Here's how the part is built. I have some questions about the finished solid (model axes, mm). A direction names the side the tool comes from. Coordinates: 2 decimals unless noted, no trailing zeros. Write each loop counter-clockwise with the first axis right and the second up, starting at its lowest first coordinate (ties: lowest second). Pieces come first, ordered by that corner, then holes.
(1) Which directions (+Z, -Z, +X, -X, +Y, -Y) give clear straight access to the entire face, cutting with the end or side of a thin tool? Please do faces 1 (the flat face through (0, 2.9, 2)), 2 (the flat face through (0, 10.9, 0)), 3 (the flat face through (-1.095, 0.937, 0.644)).
(2) Imagine slicing it at A-A, the plane x = 0. List the corners of the cut face in (y, z) for me (3 decimals).
(3) For pin 1 Ø0.8 at (x, z) = (0, 0.5) entering from -Y; pin 2 Ø2 at (y, z) = (6.5, -1) entering from +X; pin 3 Ø2 at (x, y) = (0.5, 6) entering from -Z, each with a flat end and sliding along its axis, tell me the tip position at first contact or that it passes through.
(4) Imagine slicing it at C-C, the plane x = 1.95. List the corners of the cut face in (y, z) for me, plus the area to 3 significant figures.
(5) Thinking about a two-plate mould opening in Z: for faces 4 (the cylindrical face through (-1.45, 6.72, -0.06)), 5 (the flat face through (-1.105, 0.937, -0.626)), 6 (the flat face through (0, 1, -1.27)), 7 (the flat face through (1.1, 0, 1.1)), which applies, released by +Z, released by -Z, zero draft, split by the parting line, or undercut?
(6) Imagine slicing it at B-B, the plane y = 7.5. List the corners of the cut face in (x, z) for me.
(7) Please list where these lines run through material, in increasing order: probe 1 along Y at (x, z) = (-0.2, -0.9); probe 2 along Y at (x, z) = (1.3, -1.3); probe 3 along Z at (x, y) = (0.4, 1.5).
```python
from build123d import *

# Parameters (mm, degrees)
SKETCH1_R           = 2.465
BOSS_EXTRUDE1_DEPTH = 2.9
SKETCH2_R           = 1.45
BOSS_EXTRUDE2_DEPTH = 8
CUT_EXTRUDE1_DEPTH  = 1.9
CHAMFER1_SIZE       = 0.25


with BuildPart() as part:
    # Sketch1 → Boss-Extrude1 (new body)
    with BuildSketch(Plane(origin=(0, 0, 0), x_dir=(1, 0, 0), z_dir=(0, 1, 0))):
        Circle(SKETCH1_R)
    extrude(amount=BOSS_EXTRUDE1_DEPTH)

    # Sketch2 → Boss-Extrude2 (add)
    with BuildSketch(Plane(origin=(0, 2.9, 0), x_dir=(1, 0, 0), z_dir=(0, 1, 0))):
        Circle(SKETCH2_R)
    extrude(amount=BOSS_EXTRUDE2_DEPTH)

    # Sketch3 → Cut-Extrude1 (cut)
    with BuildSketch(Plane.XZ):
        Polygon((0.733234842, -1.27), (1.466469684, 0), (0.733234842, 1.27), (-0.733234842, 1.27), (-1.466469684, 0), (-0.733234842, -1.27), align=None)
    extrude(amount=-CUT_EXTRUDE1_DEPTH, mode=Mode.SUBTRACT)

    # Chamfer1
    chamfer1_edges = [part.edges().sort_by_distance(p)[0] for p in [
        (-1.45, 10.9, 0),
    ]]
    chamfer(chamfer1_edges, length=CHAMFER1_SIZE)


solid = part.part
```
Recorded:
1. face 1: +Y
1. face 2: +Z, -Z, +X, -X, +Y
1. face 3: -Y
2. outline: (0, -2.465) - (2.9, -2.465) - (2.9, -1.45) - (10.65, -1.45) - (10.9, -1.2) - (10.9, 1.2) - (10.65, 1.45) - (2.9, 1.45) - (2.9, 2.465) - (0, 2.465) - (0, 1.27) - (1.9, 1.27) - (1.9, -1.27) - (0, -1.27) - close
3. pin 1: stops at y = 1.9
3. pin 2: stops at x = 1.45
3. pin 3: stops at z = -1.45
4. outline: (0, -1.51) - (2.9, -1.51) - (2.9, 1.51) - (0, 1.51) - close
4. area: 8.75 mm2
5. face 4: split by the parting line
5. face 5: undercut
5. face 6: undercut
5. face 7: zero draft
6. outline: circle Ø2.9 at (0, 0)
7. probe 1: y = 1.9 to 10.9
7. probe 2: y = 0 to 2.9
7. probe 3: z = -2.43 to -1.27, 1.27 to 2.43
